from build123d import *

# Parameters (mm, degrees)
SKETCH3_W               = 17.78
SKETCH3_H               = 3.175
REVOLVE2_ANGLE          = 10
CIRPATTERN1_COUNT       = 4
F_1_4_CLEARANCE_HOLE1_D = 6.7564
CIRPATTERN2_COUNT       = 4


# Read off the part's stored shape, not the designer's step: Revolve2
with BuildPart() as part:
    # Sketch3 → Revolve1 (revolve)
    with BuildSketch(Plane.XY, mode=Mode.PRIVATE) as revolve1_sk:
        with Locations((-41.91, 1.5875)):
            Rectangle(SKETCH3_W, SKETCH3_H)
    revolve(revolve1_sk.sketch.rotate(Axis((0, -0.15875, 0), (0, 1, 0)), 270), axis=Axis((0, -0.15875, 0), (0, 1, 0)))

    # Revolve2 outline → Revolve2 (revolve)
    with BuildSketch(Plane(origin=(0, 0, 0), x_dir=(-0.9961946980917455, 0, -0.0871557427476582), z_dir=(0.0871557427476582, 0, -0.9961946980917455))):
        with BuildLine():
            Line((33.02, 3.175), (50.8, 3.175))
            ThreePointArc((50.8, 3.175), (56.020671736, 19.804496878), (57.785, 37.144702343))
            Line((57.785, 37.144702343), (56.1975, 37.144702343))
            ThreePointArc((56.1975, 37.144702343), (47.732858136, 18.028274757), (33.02, 3.175))
        make_face()
    revolve2 = revolve(axis=Axis((0, 0, 0), (0, 1, 0)), revolution_arc=REVOLVE2_ANGLE)

    # CirPattern1: Revolve2 ×4 about axis
    cirpattern1_axis = Axis((0, -0.15875, 0), (0, 1, 0))
    for i in range(1, CIRPATTERN1_COUNT):
        add(revolve2.rotate(cirpattern1_axis, i * 360 / CIRPATTERN1_COUNT))

    # 1/4 Clearance Hole1 (through all)
    with Locations(Plane(origin=(0, 3.175, 0), x_dir=(1, 0, 0), z_dir=(0, 1, 0))):
        with Locations((-30.308364409, -30.308364409)):
            f_1_4_clearance_hole1 = Hole(F_1_4_CLEARANCE_HOLE1_D / 2)

    # CirPattern2: 1/4 Clearance Hole1 ×4 about axis
    cirpattern2_axis = Axis((0, 0, 0), (0, 1, 0))
    for i in range(1, CIRPATTERN2_COUNT):
        add(f_1_4_clearance_hole1.rotate(cirpattern2_axis, i * 360 / CIRPATTERN2_COUNT), mode=Mode.SUBTRACT)


solid = part.part
Geometry: final body of the model. Coordinates: model frame, mm. A direction names the side the tool comes from. Give positions to 0.01 mm unless a question says otherwise; leave off trailing zeros. Write each loop counter-clockwise with the first axis right and the second up, starting at its lowest first coordinate (ties: lowest second). Pieces come first, ordered by that corner, then holes. Notation, with made-up numbers: (56, 85) - (81, 85) arc R25 ccw to (81, 122) - close; hole circle Ø2 at (75, 19). An arc over 180 degrees is marked (long way). Return JSON: item names as keys, results as strings. Group by question number.
1) Mould query, pull axis X, two halves, no side actions, for faces 5 (the cylindrical face through (30.911, 1.61, 40.313)), 6 (the flat face through (4.35, 15.21, 49.74)), 7 (the flat face through (-49.74, 15.21, 4.35)). Classes: released by +X, released by -X, zero draft, split by the parting line, or undercut.
2) Section A-A on z = -23. Return the cut outline in (x, y) (3 decimals), plus the area to 3 significant figures.
3) Set-up query: faces 1 (the flat face through (-4.35, 15.21, -49.74)), 2 (the flat face through (49.74, 15.21, 4.35)), 3 (the flat face through (-49.74, 15.21, -4.35)), 4 (the flat face through (4.35, 15.21, -49.74)). Return all of +Z, -Z, +X, -X, +Y, -Y with unobstructed straight access to the full face (end or side cutting, diameter ignored); none if empty.
4) First-contact query: P1, Ø8, axis at x = 30.31, z = -30.31, coming from the +Y side (3 decimals); P2, Ø9, axis at x = 30.31, z = 30.31, coming from the -Y side; P3, Ø12, axis at x = 10.5, y = 9.5, coming from the -Z side. Flat tips, straight axial feed; report the tip coordinate or a pass-through.
5) Section D-D on z = -49. Return the cut outline in (x, y) (3 decimals), plus the area to 3 significant figures.
6) Section C-C on x = -38. Return the cut outline in (y, z) (3 decimals), plus the area to 3 significant figures.
7) Section B-B on x = 7.5. Return the cut outline in (y, z) (3 decimals).
8) Line query: line 1 (Y direction, x = 48, z = 6.5) (3 decimals); line 2 (X direction, y = 1, z = 0); line 3 (Z direction, x = -12, y = 2). Output: solid intervals per line, ascending.
Filled in:
{
 "1": {"face 5": "split by the parting line", "face 6": "released by +X", "face 7": "undercut"},
 "2": {"outline": "(-45.295, 0) - (-23.692, 0) - (-23.692, 3.175) - (-45.295, 3.175) - close; (23.692, 0) - (45.295, 0) - (45.295, 3.175) - (23.692, 3.175) - close", "area": "137 mm^2"},
 "3": {"face 1": "-X, +Y", "face 2": "+Z, +Y", "face 3": "-Z, +Y", "face 4": "+X, +Y"},
 "4": {"P1": "stops at y = 3.175", "P2": "stops at y = 0", "P3": "stops at z = -53.5"},
 "5": {"outline": "(-13.403, 0) - (13.403, 0) - (13.403, 3.175) - (4.287, 3.175) - (4.287, 20.269) arc R30.629 cw to (-4.287, 20.269) - (-4.287, 3.175) - (-13.403, 3.175) - close", "area": "230 mm^2"},
 "6": {"outline": "(0, -33.714) - (3.175, -33.714) - (3.175, -3.325) - (7.191, -3.325) arc R43.533 cw to (7.191, 3.325) - (3.175, 3.325) - (3.175, 33.714) - (0, 33.714) - close", "area": "240 mm^2"},
 "7": {"outline": "(0, -50.243) - (3.175, -50.243) - (3.175, -32.157) - (0, -32.157) - close; (0, 32.157) - (3.175, 32.157) - (3.175, 50.243) - (0, 50.243) - close"},
 "8": {"line 1": "y = 0 to 3.175", "line 2": "x = -50.8 to -33.02, 33.02 to 50.8", "line 3": "z = -49.36 to -30.76, 30.76 to 49.36"}
}
